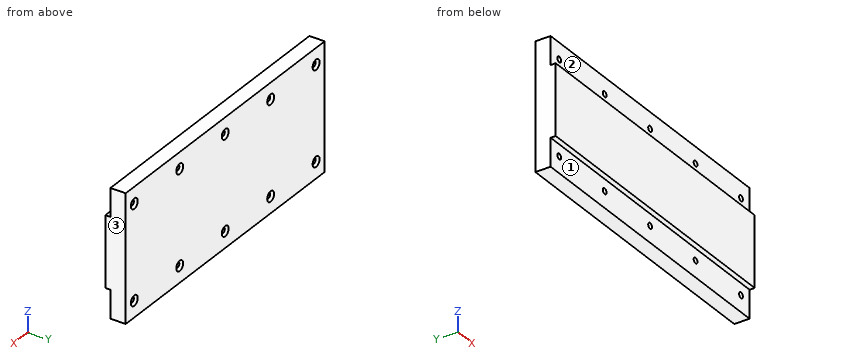
```python
from build123d import *

# Parameters (mm, degrees)
BOSS_EXTRUDE1_DEPTH                              = 290
CSK_FOR_M10_FLAT_HEAD_MACHINE_SCREW1_D           = 11
CSK_FOR_M10_FLAT_HEAD_MACHINE_SCREW1_DEPTH       = 55.695266595
CSK_FOR_M10_FLAT_HEAD_MACHINE_SCREW1_CSINK_D     = 20
CSK_FOR_M10_FLAT_HEAD_MACHINE_SCREW1_CSINK_ANGLE = 90
CSK_FOR_M10_FLAT_HEAD_MACHINE_SCREW1_TIP         = 3.304733405


with BuildPart() as part:
    # Sketch2 → Boss-Extrude1 (new, symmetric)
    with BuildSketch(Plane(origin=(0, 0, 0), x_dir=(0, 0, -1), z_dir=(1, 0, 0))):
        Polygon((-124, 0), (124, 0), (124, -30), (69, -30), (69, -40), (-69, -40), (-69, -30), (-124, -30), align=None)
    extrude(amount=BOSS_EXTRUDE1_DEPTH, both=True)

    # CSK for M10 Flat Head Machine Screw1
    with Locations(Plane(origin=(-265, 0, -92), x_dir=(0, 0, 1), z_dir=(0, 1, 0))):
        with Locations((0, 0), (0, 132.5), (0, 265), (0, 397.5), (0, 530), (184, 530), (184, 397.5), (184, 265), (184, 132.5), (184, 0)):
            CounterSinkHole(CSK_FOR_M10_FLAT_HEAD_MACHINE_SCREW1_D / 2, CSK_FOR_M10_FLAT_HEAD_MACHINE_SCREW1_CSINK_D / 2, depth=CSK_FOR_M10_FLAT_HEAD_MACHINE_SCREW1_DEPTH, counter_sink_angle=CSK_FOR_M10_FLAT_HEAD_MACHINE_SCREW1_CSINK_ANGLE)
            with Locations((0, 0, -(CSK_FOR_M10_FLAT_HEAD_MACHINE_SCREW1_DEPTH + CSK_FOR_M10_FLAT_HEAD_MACHINE_SCREW1_TIP / 2))):  # 118° drill point
                Cone(0, CSK_FOR_M10_FLAT_HEAD_MACHINE_SCREW1_D / 2, CSK_FOR_M10_FLAT_HEAD_MACHINE_SCREW1_TIP, mode=Mode.SUBTRACT)


solid = part.part
```
Here's how the part is built. I have some questions about the finished solid (model axes, mm). Face numbers are marked on the shaded views. A direction names the side the tool comes from. Give positions to 0.01 mm unless a question says otherwise; leave off trailing zeros. Write each loop counter-clockwise with the first axis right and the second up, starting at its lowest first coordinate (ties: lowest second). Pieces come first, ordered by that corner, then holes. Notation, with made-up numbers: M -22.75,-4 L -10.75,-4 A28 ccw -10.75,19 Z; hole C 82,79.5 d8. An arc over 180 degrees is marked long. Put each result on its own line as item: value. Start each with the question number.
Item 1: Will these pins go through, and if not, where does the flat tip stop? pin 1 (14.5 mm diameter, centred on x = -132.5, z = -92, fed in from +Y); pin 2 (17.5 mm diameter, centred on x = 0, z = 92, fed in from +Y); pin 3 (3 mm diameter, centred on x = 75, y = -32.5, fed in from -Z); pin 4 (2 mm diameter, centred on x = -129, z = 42, fed in from +Y).
Item 2: On a 3-axis mill with a long thin cutter (end or side, diameter ignored), from which of +Z, -Z, +X, -X, +Y, -Y can I reach the whole of each face in a straight line? I mean the marked faces 1, 2 and 3. Say none if no direction works.
Item 3: I need wall thicknesses on L1, parallel to X at y = -23.75, z = -92; L2, parallel to Z at x = 0, y = -16.75; L3, parallel to X at y = -2, z = 90.5. Which ranges of each line are inside material? Lowest first, please. Write a range as from..to.
Item 4: If we section it at A-A, the plane x = 265: Write out the boundary of the cut face in (y, z), then the cut area to 3 significant figures.
Item 5: If we section it at B-B, the plane z = 92: Count the separate pieces of the cut face and the enclosed holes in it, then the cut area to 3 significant figures.
Values:
1. pin 1: y = -2.75
1. pin 2: y = -1.25
1. pin 3: z = -69
1. pin 4: y = 0
2. face 1: -Z, +X, -X, -Y
2. face 2: +Z, +X, -X, -Y
2. face 3: +Z, -Z, +X, +Y, -Y
3. L1: -290..-270.5, -259.5..-138, -127..-5.5, 5.5..127, 138..259.5, 270.5..290
3. L2: -124..-97.5, -86.5..86.5, 97.5..124
3. L3: -290..-272.86, -257.14..-140.36, -124.64..-7.86, 7.86..124.64, 140.36..257.14, 272.86..290
4. outline: M -40,-69 L -30,-69 L -30,-86.5 L -4.5,-86.5 L 0,-82 L 0,82 L -4.5,86.5 L -30,86.5 L -30,69 L -40,69 Z; M -30,-124 L 0,-124 L 0,-102 L -4.5,-97.5 L -30,-97.5 Z; M -30,97.5 L -4.5,97.5 L 0,102 L 0,124 L -30,124 Z
4. area: 8,120 mm²
5. separate pieces: 6
5. enclosed holes: 0
5. area: 15,600 mm²
